```python
from build123d import *

# Parameters (mm, degrees)
SKETCH1_W           = 1.5
SKETCH1_H           = 11
SKETCH2_W           = 8
SKETCH2_H           = 8
BOSS_EXTRUDE1_DEPTH = 2


with BuildPart() as part:
    # Sketch1 → Revolve1 (revolve)
    with BuildSketch(Plane.XY):
        with BuildLine():
            Line((0, -5), (-1.5, -5))
            Line((-1.5, -5), (-1.5, -4.769696007))
            ThreePointArc((-1.5, -4.769696007), (-4.942088629, 0.758788496), (0, 5))
            Line((0, 5), (0, -5))
        make_face()
        with Locations((-0.75, -10.5)):
            Rectangle(SKETCH1_W, SKETCH1_H)
    revolve(axis=Axis((0, 5, 0), (0, -1, 0)))

    # Sketch2 → Boss-Extrude1 (add)
    with BuildSketch(Plane(origin=(0, -6, 0), x_dir=(-1, 0, 0), z_dir=(0, -1, 0))):
        Rectangle(SKETCH2_W, SKETCH2_H)
    extrude(amount=-BOSS_EXTRUDE1_DEPTH)


solid = part.part
```
Here's how the part is built. I have some questions about the finished solid (model axes, mm). A direction names the side the tool comes from. Give positions to 0.01 mm unless a question says otherwise; leave off trailing zeros. Loops run counter-clockwise (first coordinate to the right, second up) from the corner with the lowest first, then second, coordinate; pieces in that order, holes last. Notation, with made-up numbers: (43.25, 77) -> (77.25, 77) arc R37 ccw to (77.25, 116) -> close; hole circle Ø8 at (84.25, 72.5). An arc over 180 degrees is marked (long way). Use one line per item in the form item = value. Start each with the question number.
1) Imagine slicing it at D-D (z = -3.25). Please give me the cut outline in (x, y), then the cut area to 3 significant figures.
2) Please list where these lines run through material, in increasing order: line 1 along X through (y, z) = (-5.5, -1); line 2 along Y through (x, z) = (-3.75, 3.75); line 3 along Z through (x, y) = (0, -8.25).
3) Imagine slicing it at C-C (x = 0). Please give me the cut outline in (y, z).
4) Which directions (+Z, -Z, +X, -X, +Y, -Y) give clear straight access to the entire face, cutting with the end or side of a thin tool? Please do faces 4 (the face through (4, -5, 0)), 5 (the face through (0, -5, -4)), 6 (the face through (0, -5, 4)).
5) Thinking about a two-plate mould opening in Y: for faces 1 (the face through (2, -6, 0)), 2 (the face through (-4, -5, 0)), 3 (the face through (-2, -4, -3)), which applies, +Y half, -Y half, draft (parallel to the pull), parting line (faces both ways), or undercut?
6) For P1, Ø1.6, axis at y = -5, z = 2, coming from the -X side; P2, Ø2, axis at x = 1.5, y = -5, coming from the +Z side; P3, Ø4, axis at y = -1, z = 3.5, coming from the +X side, each with a flat end and sliding along its axis, tell me the tip position at first contact or that it passes through.
7) Imagine slicing it at A-A (z = 0). Please give me the cut outline in (x, y), then the cut area to 3 significant figures.
8) Imagine slicing it at B-B (x = 3.5). Please give me the cut outline in (y, z).
Check values:
q1.outline = (-4, -6) -> (4, -6) -> (4, -4) -> (-4, -4) -> close; circle Ø7.6 at (0, 0)
q1.area = 61.4 mm^2
q2.line_1 = -4 to 4
q2.line_2 = -6 to -4
q2.line_3 = -1.5 to 1.5
q3.outline = (-16, -1.5) -> (-6, -1.5) -> (-6, -4) -> (-4, -4) -> (-4, -3) arc R5 ccw (long way) to (-4, 3) -> (-4, 4) -> (-6, 4) -> (-6, 1.5) -> (-16, 1.5) -> close
q4.face_4 = +Z, -Z, +X, -Y
q4.face_5 = -Z, +X, -X, -Y
q4.face_6 = +Z, +X, -X, -Y
q5.face_1 = -Y half
q5.face_2 = draft
q5.face_3 = undercut
q6.P1 = -4
q6.P2 = 4
q6.P3 = 4.72
q7.outline = (-4, -6) -> (-1.5, -6) -> (-1.5, -16) -> (1.5, -16) -> (1.5, -6) -> (4, -6) -> (4, -4) -> (3, -4) arc R5 ccw (long way) to (-3, -4) -> (-4, -4) -> close
q7.area = 120 mm^2
q8.outline = (-6, -4) -> (-4, -4) -> (-4, 4) -> (-6, 4) -> close; circle Ø7.14 at (0, 0)
